Here's the drawing with two shaded views (mm, measured from the low corner). I have some questions. A direction names the side the tool comes from. Round coordinates to 2 decimals unless told otherwise and drop trailing zeros. Order: outer loops, then holes, each group sorted by start corner. A loop starts at its lowest first (then second) coordinate and runs counter-clockwise, first axis right, second up.
Q1. If I drill on line 1 (Z direction, x = 7, y = 6.75); line 2 (Z direction, x = 33.5, y = 8.5); line 3 (X direction, y = 2.75, z = 23.5), over which ranges is the centre line in solid material (lowest first)?
Q2. If we section it at C-C (x = 7): Please give me the cut outline in (y, z), plus the area to 3 significant figures.
Q3. For the marked faces 4 and 5, which set-ups out of +Z, -Z, +X, -X, +Y, -Y let a thin tool reach every point of the face, with its end or its side?
Q4. If we section it at A-A (y = 4.25): Please give me the cut outline in (x, z).
Q5. If we section it at B-B (z = 8): Please give me the cut outline in (x, y), plus the area to 3 significant figures.
Q6. We'd pull the mould along X, two halves only. Please class the marked faces 1, 2 and 3: pulls with the +X half, pulls with the -X half, needs draft (parallel to the pull), parting line crosses it, or undercut.
Q7. If we section it at D-D (y = 12.75): Please give me the cut outline in (x, z).
Q8. Will this pin go through, and if not, where does the flat tip stop? P1, Ø5, axis at x = 21, z = 28.5, coming from the -Y side.
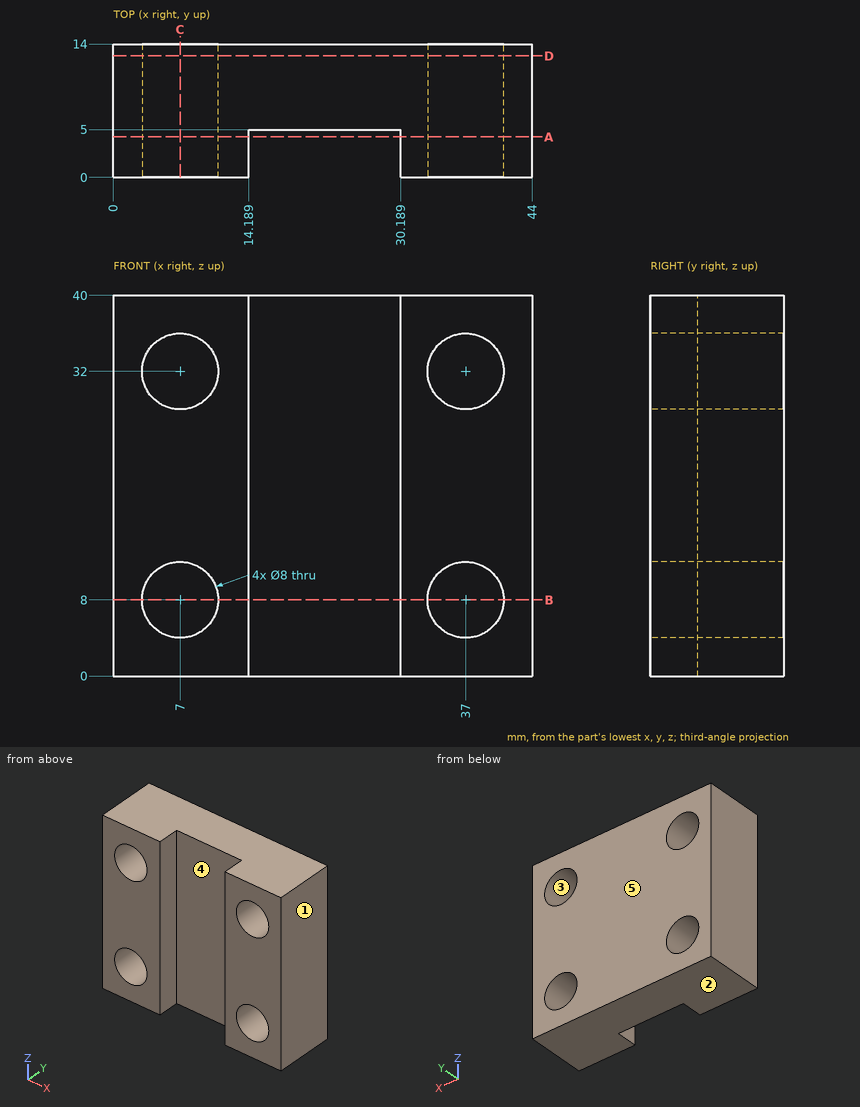
Solution:
1. line 1: z = 0 to 4, 12 to 28, 36 to 40
1. line 2: z = 0 to 6.06, 9.94 to 30.06, 33.94 to 40
1. line 3: x = 0 to 14.19, 30.19 to 44
2. outline: (0, 0) - (14, 0) - (14, 4) - (0, 4) - close; (0, 12) - (14, 12) - (14, 28) - (0, 28) - close; (0, 36) - (14, 36) - (14, 40) - (0, 40) - close
2. area: 336 mm2
3. face 4: +Z, -Z, -Y
3. face 5: +Z, -Z, +X, -X, +Y
4. outline: (0, 0) - (14.19, 0) - (14.19, 40) - (0, 40) - close; (30.19, 0) - (44, 0) - (44, 40) - (30.19, 40) - close; hole circle Ø8 at (7, 8); hole circle Ø8 at (7, 32); hole circle Ø8 at (37, 8); hole circle Ø8 at (37, 32)
5. outline: (0, 0) - (3, 0) - (3, 14) - (0, 14) - close; (11, 0) - (14.19, 0) - (14.19, 5) - (30.19, 5) - (30.19, 0) - (33, 0) - (33, 14) - (11, 14) - close; (41, 0) - (44, 0) - (44, 14) - (41, 14) - close
5. area: 312 mm2
6. face 1: pulls with the +X half
6. face 2: needs draft
6. face 3: undercut
7. outline: (0, 0) - (44, 0) - (44, 40) - (0, 40) - close; hole circle Ø8 at (7, 8); hole circle Ø8 at (7, 32); hole circle Ø8 at (37, 8); hole circle Ø8 at (37, 32)
8. P1: stops at y = 5
